Print and shaded views of the part. All mm, measured from the part's lowest x, y and z. A direction names the side the tool comes from. Coordinates: 2 decimals unless noted, no trailing zeros. Order: outer loops, then holes, each group sorted by start corner. A loop starts at its lowest first (then second) coordinate and runs counter-clockwise, first axis right, second up.
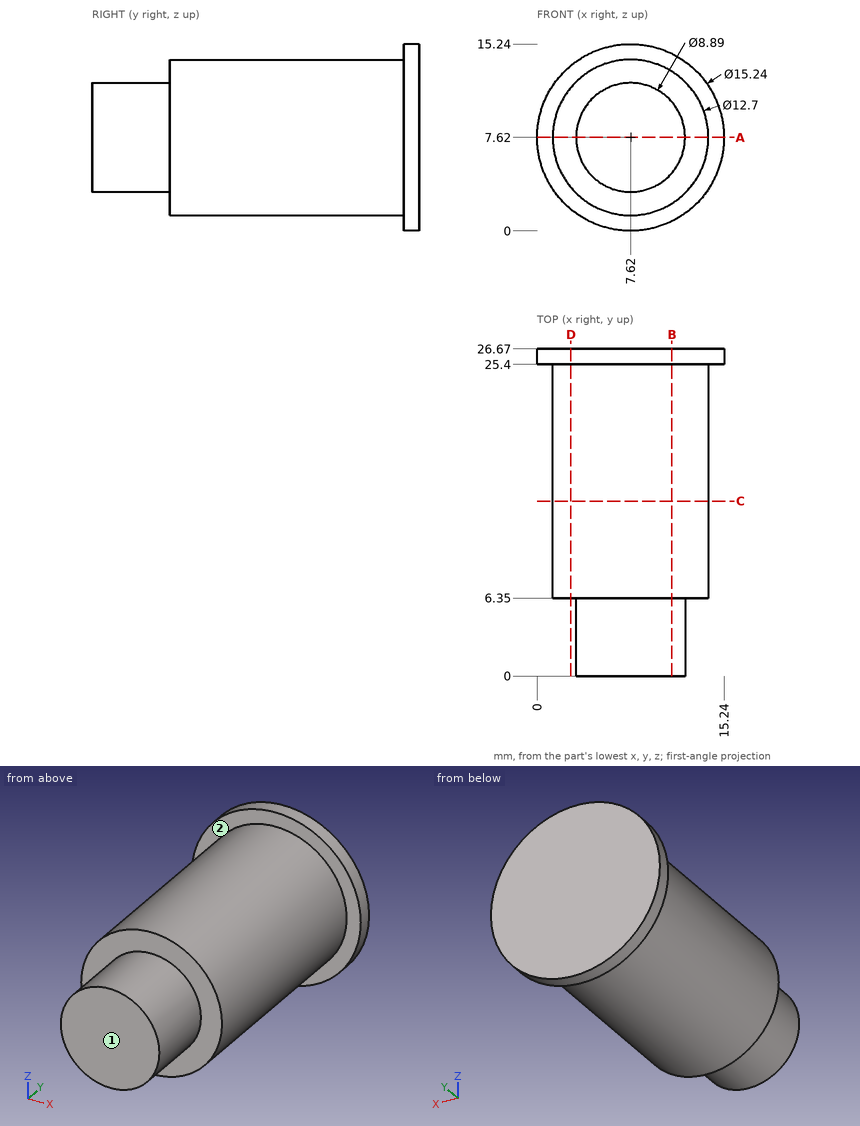
Q1. Cut at A-A, the plane z = 7.62. List the corners of the cut face in (x, y) (3 decimals).
Established:
outline: (0, 25.4) - (1.27, 25.4) - (1.27, 6.35) - (3.175, 6.35) - (3.175, 0) - (12.065, 0) - (12.065, 6.35) - (13.97, 6.35) - (13.97, 25.4) - (15.24, 25.4) - (15.24, 26.67) - (0, 26.67) - close
Q2. Which spindle directions (+Z, -Z, +X, -X, +Y, -Y) get a long thin tool onto all of the face, cutting with end or side? Do the marked faces 1 and 2. Say none if no direction does.
Established:
face 1: +Z, -Z, +X, -X, -Y
face 2: -Y
Q3. Cut at B-B, the plane x = 11. List the corners of the cut face in (y, z), plus the area to 3 significant figures.
Established:
outline: (0, 4.73) - (6.35, 4.73) - (6.35, 2.24) - (25.4, 2.24) - (25.4, 0.79) - (26.67, 0.79) - (26.67, 14.45) - (25.4, 14.45) - (25.4, 13) - (6.35, 13) - (6.35, 10.51) - (0, 10.51) - close
area: 259 mm2
Q4. Cut at D-D, the plane x = 2.75. List the corners of the cut face in (y, z) (3 decimals).
Established:
outline: (6.35, 3.545) - (25.4, 3.545) - (25.4, 1.759) - (26.67, 1.759) - (26.67, 13.481) - (25.4, 13.481) - (25.4, 11.695) - (6.35, 11.695) - close
Q5. Drop flat-ended pins along their axis: P1, Ø1, axis at x = 11, y = 21, coming from the -Z side; P2, Ø8, axis at x = 6, y = 16.5, coming from the +Z side; P3, Ø6, axis at x = 12.5, y = 23.5, coming from the -Z side. Give the stop position or say it passes through.
Established:
P1: stops at z = 1.96
P2: stops at z = 13.97
P3: stops at z = 0.44
Q6. Probe line 1 (Y direction, x = 4.25, z = 1.75); line 2 (Y direction, x = 8, z = 2); line 3 (Z direction, x = 11.75, y = 7.75). List the from-to ranges inside material, lowest first.
Established:
line 1: y = 25.4 to 26.67
line 2: y = 6.35 to 26.67
line 3: z = 2.8 to 12.44
Q7. Cut at C-C, the plane y = 14.25. List the corners of the cut face in (x, z), plus the area to 3 significant figures.
Established:
outline: circle Ø12.7 at (7.62, 7.62)
area: 127 mm2
